Autodesk Inventor part; units mm, degrees
ref_plane "YZ Plane" through (0, 0, 0) normal (1, 0, 0) x (0, 1, 0)
ref_plane "XZ Plane" through (0, 0, 0) normal (0, 1, 0) x (-1, 0, 0)
ref_plane "XY Plane" through (0, 0, 0) normal (0, 0, 1) x (1, 0, 0)
sketch "Sketch1" plane through (0, 0, 0) normal (0, 0, 1) x (1, 0, 0)
  line L0 (40, -100) -> (-40, -100)
  line L1 (-40, -100) -> (-40, 100)
  line L2 (-40, 100) -> (40, 100)
  line L3 (40, 100) -> (40, -100)
  line L4 (40, 100) -> (-40, -100) construction
  point P0 (0, 0)
  point P1 (0, 0)
  dimension "d1" = 200
  dimension "d2" = 80
extrude "Plate1" add sketch "Sketch1" along normal blind 2
sketch "Sketch5" plane through (0, 0, 0) normal (0, 0, 1) x (1, 0, 0)
  circle A0 centre (-32, 92) radius 3
  circle A1 centre (-32, 4) radius 3
  line L0 (-40, -100) -> (-40, 100)
  line L1 (40, -100) -> (-40, -100)
  line L2 (40, 100) -> (40, -100)
  line L3 (-40, 100) -> (40, 100)
  line L4 (-32, 92) -> (-32, 77) construction
  line L5 (-35, 92) -> (-35, 77)
  line L6 (-29, 77) -> (-29, 92)
  arc A2 (-29, 92) -> (-35, 92) centre (-32, 92) ccw
  arc A3 (-35, 77) -> (-29, 77) centre (-32, 77) ccw
  line L7 (-32, 4) -> (-32, -11) construction
  line L8 (-35, 4) -> (-35, -11)
  line L9 (-29, -11) -> (-29, 4)
  arc A4 (-29, 4) -> (-35, 4) centre (-32, 4) ccw
  arc A5 (-35, -11) -> (-29, -11) centre (-32, -11) ccw
  point P0 (0, 0)
  point P1 (-32, 84.5)
  point P2 (-32, -3.5)
  point P3 (-29, 4)
  dimension "d33" = 88
  dimension "d34" = 6
  dimension "d35" = 8
  dimension "d36" = 8
  dimension "d50" = 15
extrude "Cut1" cut sketch "Sketch5" along normal blind 2 contours A0 | L6 A3 L5 A0 | A1 | L9 A5 L8 A1
sketch "Sketch6" plane through (38, 100, 2) normal (1, 0, 0) x (0, 1, 0)
  line L0 (-200, 0) -> (0, 0)
  line L1 (0, 0) -> (0, 30)
  line L2 (0, 30) -> (-200, 30)
  line L3 (-200, 30) -> (-200, 0)
edge flange "Flange2" height 30 angle 90 thickness 2 bend radius 2 thickness toward (1, 0, 0) relief tear relief width 2 relief depth 1 edges at (40, 0, 2) wall of the first edge with corners at (38, -100, 2) (38, 100, 2) (38, 100, -28) (38, -100, -28)
bend "Bend2"
corner "Corner2"
fillet "Corner Round1" radius 6 4 edges at (-40, 100, 1) (39, -100, -28) (39, 100, -28) (-40, -100, 1)
equation "\"d36\" = d35"
equation "\"d37\" = Thickness"
equation "\"d0\" = Thickness"
equation "\"d39\" = BendReliefWidth"
equation "\"d40\" = BendReliefDepth"
equation "\"d41\" = MinimumRemnant"
equation "\"d42\" = TransitionRadius"
equation "\"d45\" = BendRadius"
equation "\"d46\" = CornerReliefSize"
equation "\"d47\" = GapSize"
equation "\"d48\" = JacobiRadiusSize"
equation "\"BendRadius\" = Thickness"
equation "\"BendReliefWidth\" = Thickness"
equation "\"BendReliefDepth\" = 0.5 * Thickness"
equation "\"CornerReliefSize\" = 4 * Thickness"
equation "\"MinimumRemnant\" = 2 * Thickness"
equation "\"TransitionRadius\" = BendRadius"
equation "\"JacobiRadiusSize\" = BendRadius"
equation "\"GapSize\" = Thickness"
properties part number "GNH 017  Pulse compensator" material "Stainless Steel"
Model file for the job. Use its own axes, mm. A direction names the side the tool comes from. Coordinates: 2 decimals unless noted, no trailing zeros. Order: outer loops, then holes, each group sorted by start corner. A loop starts at its lowest first (then second) coordinate and runs counter-clockwise, first axis right, second up. Notation, with made-up numbers: (29, 88) -> (65, 88) arc R4 ccw to (65, 94) -> close; hole circle Ø10 at (53, 70.5). An arc over 180 degrees is marked (long way). Answer as a JSON object with one key per item and string values. Group by question number.
1) Cut at D-D, the plane z = -10.25. Write the cut outline in (x, y).
2) Cut at B-B, the plane y = -62. Write the cut outline in (x, z), then the cut area to 3 significant figures.
3) Drill centre lines: L1, parallel to X at y = -14.5, z = -13.25; L2, parallel to Z at x = 9, y = 81.5. Where is each one in solid material? Low to high.
4) Cut at A-A, the plane x = -32. Write the cut outline in (y, z).
5) Which spindle directions (+Z, -Z, +X, -X, +Y, -Y) get a long thin tool onto all of the face, cutting with end or side? Do faces 1 (the face through (-38.289, -98.196, 1.014)), 2 (the face through (-3, 1, 0)). Say none if no direction does.
6) Flat gauge pins, fed straight in: pin 1 (1 mm diameter, centred on y = 87, z = 1.5, fed in from +X); pin 2 (8 mm diameter, centred on y = 25.5, z = -10, fed in from -X); pin 3 (10 mm diameter, centred on x = 13.5, z = -8.5, fed in from -Y); pin 4 (2 mm diameter, centred on y = -4, z = 1, fed in from +X). Where does each tip first touch, or does it go through?
7) Cut at C-C, the plane x = 3.5. Write the cut outline in (y, z).
Check values:
{
 "1": {"outline": "(38, -100) -> (40, -100) -> (40, 100) -> (38, 100) -> close"},
 "2": {"outline": "(-40, 0) -> (36, 0) arc R2 cw to (38, -2) -> (38, -28) -> (40, -28) -> (40, -2) arc R4 ccw to (36, 2) -> (-40, 2) -> close", "area": "213 mm²"},
 "3": {"L1": "x = 38 to 40", "L2": "z = 0 to 2"},
 "4": {"outline": "(-100, 0) -> (-14, 0) -> (-14, 2) -> (-100, 2) -> close; (7, 0) -> (74, 0) -> (74, 2) -> (7, 2) -> close; (95, 0) -> (100, 0) -> (100, 2) -> (95, 2) -> close"},
 "5": {"face 1": "+Z, -Z, -X, -Y", "face 2": "-Z, -X, +Y, -Y"},
 "6": {"pin 1": "stops at x = 38.65", "pin 2": "stops at x = 38", "pin 3": "passes through", "pin 4": "stops at x = 39.46"},
 "7": {"outline": "(-100, 0) -> (100, 0) -> (100, 2) -> (-100, 2) -> close"}
}
